Answer from the drawing. Dimensions are ordinates in mm from the lowest x, y and z of the part. Round coordinates to 2 decimals unless told otherwise and drop trailing zeros. Write each loop counter-clockwise with the first axis right and the second up, starting at its lowest first coordinate (ties: lowest second). Pieces come first, ordered by that corner, then holes. Notation, with made-up numbers: (73, 75) - (86, 75) arc R17 cw to (86, 86) - close; hole circle Ø8 at (18.25, -32.75). An arc over 180 degrees is marked (long way). Answer as a JSON object with one key per item and string values.
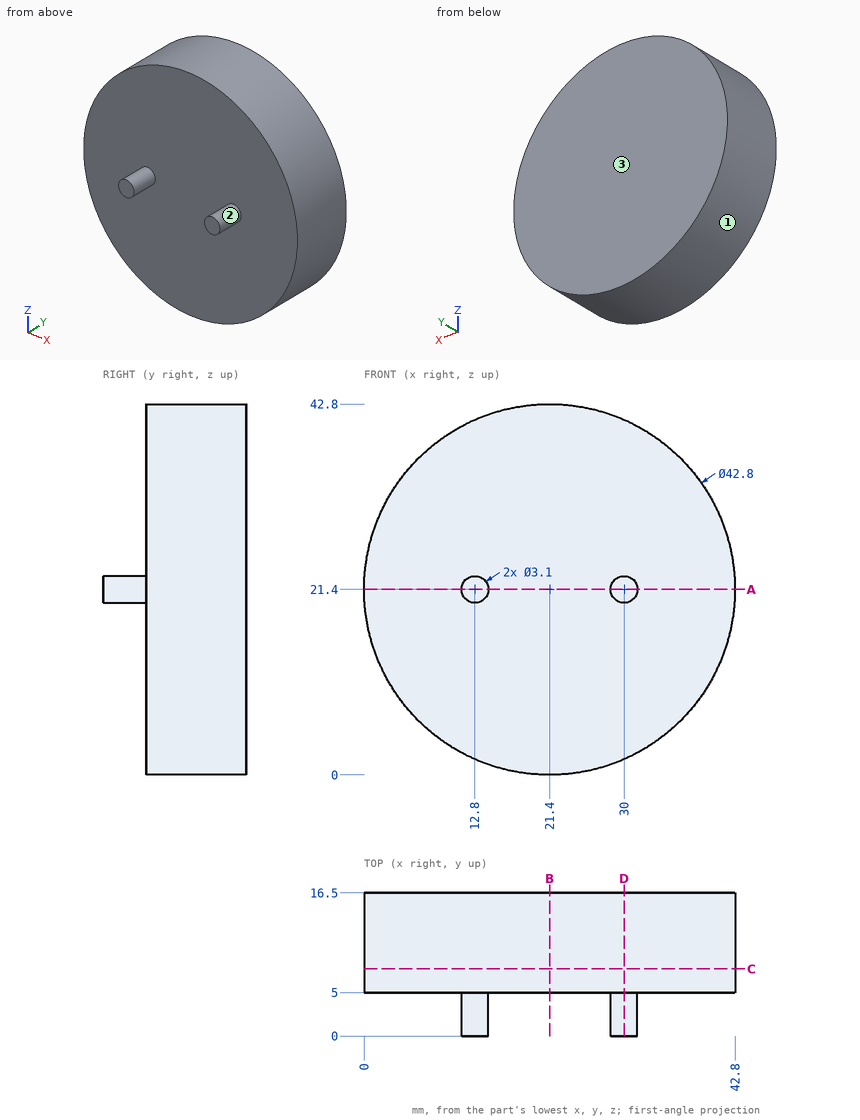
Item 1: A cutting plane is placed at C-C (y = 7.75). Write down the section's boundary in (x, z), and give its area (3 significant figures).
Results found:
{"outline": "circle Ø42.8 at (21.4, 21.4)", "area": "1,440 mm²"}
Item 2: A cutting plane is placed at D-D (x = 30). Write down the section's boundary in (y, z).
Results found:
{"outline": "(0, 19.85) - (5, 19.85) - (5, 1.8) - (16.5, 1.8) - (16.5, 41) - (5, 41) - (5, 22.95) - (0, 22.95) - close"}
Item 3: A cutting plane is placed at B-B (x = 21.4). Write down the section's boundary in (y, z), and give its area (3 significant figures).
Results found:
{"outline": "(5, 0) - (16.5, 0) - (16.5, 42.8) - (5, 42.8) - close", "area": "492 mm²"}
Item 4: Each of these flat-tipped pins is pushed along its axis until it touches: P1, Ø1, axis at x = 4.5, z = 6.5, coming from the -Y side; P2, Ø3, axis at x = 25, y = 12.5, coming from the +Z side; P3, Ø1, axis at y = 9, z = 14, coming from the -X side; P4, Ø5, axis at x = 24.5, y = 5, coming from the -Z side. Where does it stop, or does it pass through?
Results found:
{"P1": "through", "P2": "z = 42.7", "P3": "x = 1.14", "P4": "z = 0.01"}
Item 5: Determine the mould class of the marked faces 1, 2 and 3 for opening direction X: pulls with the +X half, pulls with the -X half, needs draft (parallel to the pull), parting line crosses it, or undercut.
Results found:
{"face 1": "parting line crosses it", "face 2": "undercut", "face 3": "needs draft"}
Item 6: A cutting plane is placed at A-A (z = 21.4). Write down the section's boundary in (x, y).
Results found:
{"outline": "(0, 5) - (11.25, 5) - (11.25, 0) - (14.35, 0) - (14.35, 5) - (28.45, 5) - (28.45, 0) - (31.55, 0) - (31.55, 5) - (42.8, 5) - (42.8, 16.5) - (0, 16.5) - close"}
Item 7: Consider line 1 along Y through (x, z) = (16.5, 8); line 2 along Z through (x, y) = (21.5, 14); line 3 along X through (y, z) = (10, 31.5). Determine where each line is inside the solid, lowest interval first.
Results found:
{"line 1": "5 to 16.5", "line 2": "0 to 42.8", "line 3": "2.53 to 40.27"}
